Can you work these out from the model? Positions are in its coordinate system, mm. Round coordinates to 2 decimals unless told otherwise and drop trailing zeros.
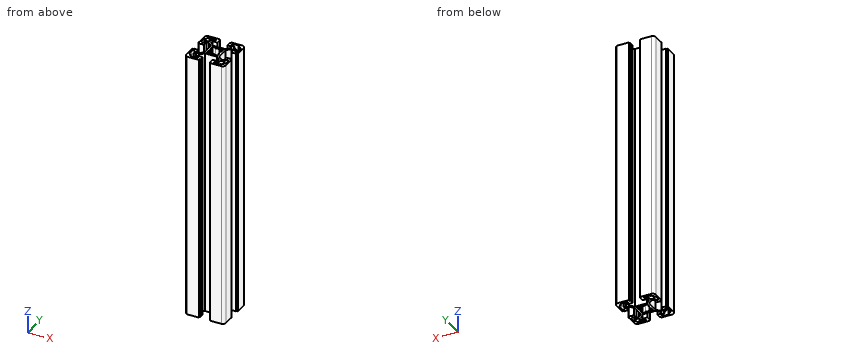
from build123d import *

# Parameters (mm, degrees)
EXTRUDE1_DEPTH = 270


with BuildPart() as part:
    # Sketch1 → Extrude1 (new body)
    with BuildSketch(Plane.XY):
        with BuildLine():
            Line((5.8, -20), (17, -20))
            ThreePointArc((17, -20), (19.121320344, -19.121320344), (20, -17))
            Line((20, -17), (20, -5.8))
            Line((20, -5.8), (18.5, -5.8))
            Line((18.5, -5.8), (18.5, -5))
            Line((18.5, -5), (14, -5))
            Line((14, -5), (14, -10.05))
            Line((14, -10.05), (11.464213562, -10.05))
            Line((11.464213562, -10.05), (7.5, -6.085786438))
            Line((7.5, -6.085786438), (7.5, 6.085786438))
            Line((7.5, 6.085786438), (11.464213562, 10.05))
            Line((11.464213562, 10.05), (14, 10.05))
            Line((14, 10.05), (14, 5))
            Line((14, 5), (18.5, 5))
            Line((18.5, 5), (18.5, 5.8))
            Line((18.5, 5.8), (20, 5.8))
            Line((20, 5.8), (20, 17))
            ThreePointArc((20, 17), (19.121320344, 19.121320344), (17, 20))
            Line((17, 20), (5.8, 20))
            Line((5.8, 20), (5.8, 18.5))
            Line((5.8, 18.5), (5, 18.5))
            Line((5, 18.5), (5, 14))
            Line((5, 14), (10.05, 14))
            Line((10.05, 14), (10.05, 11.464213562))
            Line((10.05, 11.464213562), (6.085786438, 7.5))
            Line((6.085786438, 7.5), (-6.085786438, 7.5))
            Line((-6.085786438, 7.5), (-10.05, 11.464213562))
            Line((-10.05, 11.464213562), (-10.05, 14))
            Line((-10.05, 14), (-5, 14))
            Line((-5, 14), (-5, 18.5))
            Line((-5, 18.5), (-5.8, 18.5))
            Line((-5.8, 18.5), (-5.8, 20))
            Line((-5.8, 20), (-17, 20))
            ThreePointArc((-17, 20), (-19.121320344, 19.121320344), (-20, 17))
            Line((-20, 17), (-20, 5.8))
            Line((-20, 5.8), (-18.5, 5.8))
            Line((-18.5, 5.8), (-18.5, 5))
            Line((-18.5, 5), (-14, 5))
            Line((-14, 5), (-14, 10.05))
            Line((-14, 10.05), (-11.464213562, 10.05))
            Line((-11.464213562, 10.05), (-7.5, 6.085786438))
            Line((-7.5, 6.085786438), (-7.5, -6.085786438))
            Line((-7.5, -6.085786438), (-11.464213562, -10.05))
            Line((-11.464213562, -10.05), (-14, -10.05))
            Line((-14, -10.05), (-14, -5))
            Line((-14, -5), (-18.5, -5))
            Line((-18.5, -5), (-18.5, -5.8))
            Line((-18.5, -5.8), (-20, -5.8))
            Line((-20, -5.8), (-20, -17))
            ThreePointArc((-20, -17), (-19.121320344, -19.121320344), (-17, -20))
            Line((-17, -20), (-5.8, -20))
            Line((-5.8, -20), (-5.8, -18.5))
            Line((-5.8, -18.5), (-5, -18.5))
            Line((-5, -18.5), (-5, -14))
            Line((-5, -14), (-10.05, -14))
            Line((-10.05, -14), (-10.05, -11.464213562))
            Line((-10.05, -11.464213562), (-6.085786438, -7.5))
            Line((-6.085786438, -7.5), (6.085786438, -7.5))
            Line((6.085786438, -7.5), (10.05, -11.464213562))
            Line((10.05, -11.464213562), (10.05, -14))
            Line((10.05, -14), (5, -14))
            Line((5, -14), (5, -18.5))
            Line((5, -18.5), (5.8, -18.5))
            Line((5.8, -18.5), (5.8, -20))
        make_face()
        with BuildLine():
            Line((14.5, -18.5), (9.5, -18.5))
            ThreePointArc((9.5, -18.5), (8, -17), (9.5, -15.5))
            Line((9.5, -15.5), (11.75, -15.5))
            Line((11.75, -15.5), (11.75, -14.5))
            ThreePointArc((11.75, -14.5), (12.555456352, -12.555456352), (14.5, -11.75))
            Line((14.5, -11.75), (15.5, -11.75))
            Line((15.5, -11.75), (15.5, -9.5))
            ThreePointArc((15.5, -9.5), (17, -8), (18.5, -9.5))
            Line((18.5, -9.5), (18.5, -14.5))
            Line((18.5, -14.5), (17.25, -14.5))
            ThreePointArc((17.25, -14.5), (16.444543648, -16.444543648), (14.5, -17.25))
            Line((14.5, -17.25), (14.5, -18.5))
        make_face(mode=Mode.SUBTRACT)
        with BuildLine():
            Line((18.5, 14.5), (17.25, 14.5))
            ThreePointArc((17.25, 14.5), (16.444543648, 16.444543648), (14.5, 17.25))
            Line((14.5, 17.25), (14.5, 18.5))
            Line((14.5, 18.5), (9.5, 18.5))
            ThreePointArc((9.5, 18.5), (8, 17), (9.5, 15.5))
            Line((9.5, 15.5), (11.75, 15.5))
            Line((11.75, 15.5), (11.75, 14.5))
            ThreePointArc((11.75, 14.5), (12.555456352, 12.555456352), (14.5, 11.75))
            Line((14.5, 11.75), (15.5, 11.75))
            Line((15.5, 11.75), (15.5, 9.5))
            ThreePointArc((15.5, 9.5), (17, 8), (18.5, 9.5))
            Line((18.5, 9.5), (18.5, 14.5))
        make_face(mode=Mode.SUBTRACT)
        with BuildLine():
            Line((5.5, 5.5), (2.397915762, 5.5))
            Line((2.397915762, 5.5), (1.998263135, 4.583333333))
            ThreePointArc((1.998263135, 4.583333333), (0, 5), (-1.998263135, 4.583333333))
            Line((-1.998263135, 4.583333333), (-2.397915762, 5.5))
            Line((-2.397915762, 5.5), (-5.5, 5.5))
            Line((-5.5, 5.5), (-5.5, 2.397915762))
            Line((-5.5, 2.397915762), (-4.583333333, 1.998263135))
            ThreePointArc((-4.583333333, 1.998263135), (-5, 0), (-4.583333333, -1.998263135))
            Line((-4.583333333, -1.998263135), (-5.5, -2.397915762))
            Line((-5.5, -2.397915762), (-5.5, -5.5))
            Line((-5.5, -5.5), (-2.397915762, -5.5))
            Line((-2.397915762, -5.5), (-1.998263135, -4.583333333))
            ThreePointArc((-1.998263135, -4.583333333), (0, -5), (1.998263135, -4.583333333))
            Line((1.998263135, -4.583333333), (2.397915762, -5.5))
            Line((2.397915762, -5.5), (5.5, -5.5))
            Line((5.5, -5.5), (5.5, -2.397915762))
            Line((5.5, -2.397915762), (4.583333333, -1.998263135))
            ThreePointArc((4.583333333, -1.998263135), (5, 0), (4.583333333, 1.998263135))
            Line((4.583333333, 1.998263135), (5.5, 2.397915762))
            Line((5.5, 2.397915762), (5.5, 5.5))
        make_face(mode=Mode.SUBTRACT)
        with BuildLine():
            Line((-18.5, -14.5), (-17.25, -14.5))
            ThreePointArc((-17.25, -14.5), (-16.444543648, -16.444543648), (-14.5, -17.25))
            Line((-14.5, -17.25), (-14.5, -18.5))
            Line((-14.5, -18.5), (-9.5, -18.5))
            ThreePointArc((-9.5, -18.5), (-8, -17), (-9.5, -15.5))
            Line((-9.5, -15.5), (-11.75, -15.5))
            Line((-11.75, -15.5), (-11.75, -14.5))
            ThreePointArc((-11.75, -14.5), (-12.555456352, -12.555456352), (-14.5, -11.75))
            Line((-14.5, -11.75), (-15.5, -11.75))
            Line((-15.5, -11.75), (-15.5, -9.5))
            ThreePointArc((-15.5, -9.5), (-17, -8), (-18.5, -9.5))
            Line((-18.5, -9.5), (-18.5, -14.5))
        make_face(mode=Mode.SUBTRACT)
        with BuildLine():
            Line((-14.5, 18.5), (-9.5, 18.5))
            ThreePointArc((-9.5, 18.5), (-8, 17), (-9.5, 15.5))
            Line((-9.5, 15.5), (-11.75, 15.5))
            Line((-11.75, 15.5), (-11.75, 14.5))
            ThreePointArc((-11.75, 14.5), (-12.555456352, 12.555456352), (-14.5, 11.75))
            Line((-14.5, 11.75), (-15.5, 11.75))
            Line((-15.5, 11.75), (-15.5, 9.5))
            ThreePointArc((-15.5, 9.5), (-17, 8), (-18.5, 9.5))
            Line((-18.5, 9.5), (-18.5, 14.5))
            Line((-18.5, 14.5), (-17.25, 14.5))
            ThreePointArc((-17.25, 14.5), (-16.444543648, 16.444543648), (-14.5, 17.25))
            Line((-14.5, 17.25), (-14.5, 18.5))
        make_face(mode=Mode.SUBTRACT)
    extrude(amount=EXTRUDE1_DEPTH)


solid = part.part
(1) If I drill on line 1 (Y direction, x = -15, z = 102); line 2 (Y direction, x = 16.5, z = 157.5); line 3 (X direction, y = -9, z = 167.5), over which ranges is the centre line in solid material (lowest first)?
Worked answers:
line 1: y = -20 to -17.2, -11.75 to -5, 5 to 11.75, 17.2 to 20
line 2: y = -20 to -16.39, -8.09 to -5, 5 to 8.09, 16.39 to 20
line 3: x = -20 to -18.41, -15.59 to -14, -10.41 to -7.59, 7.59 to 10.41, 14 to 15.59, 18.41 to 20
(2) Will these pins go through, and if not, where does the flat tip stop? P1, Ø1.4, axis at y = 18, z = 109, coming from the -X side; P2, Ø2.5, axis at y = -4.5, z = 172, coming from the +X side; P3, Ø12, axis at x = 15.5, y = -15.5, coming from the +Z side; P4, Ø1, axis at x = 18, z = 134, coming from the +Y side.
Worked answers:
P1: stops at x = -19.98
P2: stops at x = 18.5
P3: stops at z = 270
P4: stops at y = 19.96
(3) If we section it at A-A, the plane z = 163.5: State how many separate pieces and enclosed holes the cut face has, then the cut area to 3 significant figures.
Worked answers:
separate pieces: 1
enclosed holes: 5
area: 556 mm2
